```python
from build123d import *
from build123d.topology import SkipClean

# Parameters (mm, degrees)
ESBO_O1_R                = 55
RESSALTO_EXTRUS_O1_DEPTH = 6
ESBO_O2_R                = 10
RESSALTO_EXTRUS_O2_DEPTH = 8
FILETE3_R                = 8
ESBO_O3_R                = 2.575
CORTE_EXTRUS_O1_DEPTH    = 79.192071209
PADR_OCIRCULAR1_COUNT    = 12
CORTE_EXTRUS_O2_DEPTH    = 79.192071209
ESBO_O5_R                = 2.575
CORTE_EXTRUS_O3_DEPTH    = 79.192071209
PADR_OCIRCULAR2_COUNT    = 12
ESBO_O6_R                = 2.575
CORTE_EXTRUS_O4_DEPTH    = 79.192071209
PADR_OCIRCULAR3_COUNT    = 12


with BuildPart() as part:
    # Esboço1 → Ressalto-extrusão1 (new body)
    with BuildSketch(Plane.XY):
        Circle(ESBO_O1_R)
    extrude(amount=RESSALTO_EXTRUS_O1_DEPTH)

    # Esboço2 → Ressalto-extrusão2 (add)
    with BuildSketch(Plane.XY.offset(6)):
        Circle(ESBO_O2_R)
        with BuildLine():
            Line((-2.24624687, 2.1), (2.24624687, 2.1))
            ThreePointArc((2.24624687, 2.1), (0, -3.075), (-2.24624687, 2.1))
        make_face(mode=Mode.SUBTRACT)
    extrude(amount=RESSALTO_EXTRUS_O2_DEPTH)

    # Filete3
    filete3_edges = [part.edges().sort_by_distance(p)[0] for p in [
        (-10, 0, 6),
    ]]
    fillet(filete3_edges, radius=FILETE3_R - 0.0001)  # a hair under: the kernel refuses the full size

    # Esboço3 → Corte-extrusão1 (cut, through all)
    with BuildSketch(Plane.XY.offset(6)):
        with Locations((0, 48)):
            Circle(ESBO_O3_R)
    corte_extrus_o1 = extrude(amount=-CORTE_EXTRUS_O1_DEPTH, mode=Mode.SUBTRACT)

    # PadrãoCircular1: Corte-extrusão1 ×12 about axis
    padr_ocircular1_axis = Axis((0, 0, 0), (0, 0, 1))
    for i in range(1, PADR_OCIRCULAR1_COUNT):
        add(corte_extrus_o1.rotate(padr_ocircular1_axis, i * 360 / PADR_OCIRCULAR1_COUNT), mode=Mode.SUBTRACT)

    # Esboço4 → Corte-extrusão2 (cut, through all)
    with SkipClean():  # the faces are left unmerged after this step: merging them gives an invalid solid
        with BuildSketch(Plane.XY.offset(6)):
            with BuildLine():
                Line((2.24624687, 2.1), (-2.24624687, 2.1))
                ThreePointArc((-2.24624687, 2.1), (0, -3.075), (2.24624687, 2.1))
            make_face()
        extrude(amount=-CORTE_EXTRUS_O2_DEPTH, mode=Mode.SUBTRACT)

    # Esboço5 → Corte-extrusão3 (cut, through all)
    with SkipClean():  # the faces are left unmerged after this step: merging them gives an invalid solid
        with BuildSketch(Plane.XY.offset(6)):
            with Locations((9.835123714, 36.705181399)):
                Circle(ESBO_O5_R)
        corte_extrus_o3 = extrude(amount=-CORTE_EXTRUS_O3_DEPTH, mode=Mode.SUBTRACT)

    # PadrãoCircular2: Corte-extrusão3 ×12 about axis
    with SkipClean():  # the faces are left unmerged after this step: merging them gives an invalid solid
        padr_ocircular2_axis = Axis((0, 0, 0), (0, 0, 1))
        for i in range(1, PADR_OCIRCULAR2_COUNT):
            add(corte_extrus_o3.rotate(padr_ocircular2_axis, i * 360 / PADR_OCIRCULAR2_COUNT), mode=Mode.SUBTRACT)

    # Esboço6 → Corte-extrusão4 (cut, through all)
    with SkipClean():  # the faces are left unmerged after this step: merging them gives an invalid solid
        with BuildSketch(Plane.XY.offset(6)):
            with Locations((0, 28)):
                Circle(ESBO_O6_R)
        corte_extrus_o4 = extrude(amount=-CORTE_EXTRUS_O4_DEPTH, mode=Mode.SUBTRACT)

    # PadrãoCircular3: Corte-extrusão4 ×12 about axis
    with SkipClean():  # the faces are left unmerged after this step: merging them gives an invalid solid
        padr_ocircular3_axis = Axis((0, 0, 0), (0, 0, 1))
        for i in range(1, PADR_OCIRCULAR3_COUNT):
            add(corte_extrus_o4.rotate(padr_ocircular3_axis, i * 360 / PADR_OCIRCULAR3_COUNT), mode=Mode.SUBTRACT)


solid = part.part
```
Check sheet for the modelled part. Datum: model origin and axes. Units: mm. Give positions to 0.01 mm unless a question says otherwise; leave off trailing zeros. Loops run counter-clockwise (first coordinate to the right, second up) from the corner with the lowest first, then second, coordinate; pieces in that order, holes last. Notation, with made-up numbers: (-20.5, 51) - (13.5, 51) arc R17 ccw to (13.5, 71) - close; hole circle Ø4 at (36, 22.5). An arc over 180 degrees is marked (long way). One line per question, with ' | ' between items. Start each with the question number.
1. Draft check along X on faces 1 (the flat face through (-13, 13, 6)), 2 (the cylindrical face through (-24.99, 39.19, 3.04)). Enter one of: released by +X, released by -X, zero draft, split by the parting line, or undercut.
2. Cross-section at D-D, the plane z = 7.5. Enter the section's corners in (x, y) (3 decimals), plus the area to 3 significant figures.
3. Cross-section at B-B, the plane x = 48. Enter the section's corners in (y, z) (3 decimals), plus the area to 3 significant figures.
4. Material ranges on line 1 along Y through (x, z) = (0, 2.6) (3 decimals); line 2 along Y through (x, z) = (37.5, 3); line 3 along Y through (x, z) = (-48, 2.4) (3 decimals), recorded low to high. Write a range as [from, to].
5. Cross-section at A-A, the plane y = 0. Give the number of separate pieces and of enclosed holes in the cut face, plus the area to 3 significant figures.
6. Gauge pin test, flat ends, axial feed: pin 1 Ø5 at (x, z) = (-4, 10.5) entering from -Y; pin 2 Ø6.5 at (x, y) = (-48, 0) entering from +Z; pin 3 Ø4 at (x, y) = (24, 41.57) entering from +Z; pin 4 Ø3.5 at (x, z) = (0, 3) entering from -Y. Record the tip position at first contact, or that the pin passes through.
Check result:
1) face 1: zero draft | face 2: undercut
2) outline: circle Ø26.672 at (0, 0); hole (-2.246, 2.1) arc R3.075 ccw (long way) to (2.246, 2.1) - close | area: 532 mm2
3) outline: (-26.851, 0) - (-2.575, 0) - (-2.575, 6) - (-26.851, 6) - close; (2.575, 0) - (26.851, 0) - (26.851, 6) - (2.575, 6) - close | area: 291 mm2
4) line 1: y = [-55, -50.575], [-45.425, -30.575], [-25.425, -3.075], [2.1, 25.425], [30.575, 45.425], [50.575, 55] | line 2: y = [-40.23, -12.28], [-7.39, 7.39], [12.28, 40.23] | line 3: y = [-26.851, -2.575], [2.575, 26.851]
5) separate pieces: 6 | enclosed holes: 0 | area: 638 mm2
6) pin 1: stops at y = -12.16 | pin 2: stops at z = 6 | pin 3: passes through | pin 4: stops at y = -55
